Autodesk Inventor part; units mm, degrees
ref_plane "YZ Plane" through (0, 0, 0) normal (1, 0, 0) x (0, 1, 0)
ref_plane "XZ Plane" through (0, 0, 0) normal (0, 1, 0) x (-1, 0, 0)
ref_plane "XY Plane" through (0, 0, 0) normal (0, 0, 1) x (1, 0, 0)
sketch "Náčrt1" plane through (0, 0, 0) normal (0, 0, 1) x (1, 0, 0)
  line L0 (0, 0) -> (50, 0)
  line L1 (50, 0) -> (50, -50)
  line L2 (50, -50) -> (0, -50)
  line L3 (0, -50) -> (0, 0)
  dimension "d0" = 50
  dimension "d1" = 50
extrude "Vysunutí1" add sketch "Náčrt1" against normal blind 50
sketch "Náčrt2" plane through (0, 0, 0) normal (0, 1, 0) x (1, 0, 0)
  line L0 (12, 12) -> (38, 12)
  line L1 (38, 12) -> (38, 50)
  line L2 (38, 50) -> (12, 50)
  line L3 (12, 50) -> (12, 12)
  line L4 (0, 50) -> (50, 50)
  line L5 (0, 0) -> (0, 50)
  dimension "d4" = 12
  dimension "d5" = 26
  dimension "d6" = 38
extrude "Vysunutí2" cut sketch "Náčrt2" against normal blind 50
sketch "Náčrt3" plane through (50, -50, 0) normal (1, 0, 0) x (0, 0, -1)
  line L0 (12, 50) -> (37, 50)
  line L1 (37, 50) -> (37, 44)
  line L2 (37, 44) -> (12, 44)
  line L3 (12, 44) -> (12, 50)
  line L4 (0, 50) -> (50, 50)
  line L5 (0, 0) -> (0, 50)
  point P0 (37, 47)
  point P1 (12, 47)
  dimension "d9" = 12
  dimension "d10" = 25
  dimension "d11" = 6
extrude "Vysunutí3" cut sketch "Náčrt3" against normal blind 50
sketch "Náčrt4" plane through (50, -50, 0) normal (1, 0, 0) x (0, 0, -1)
  line L0 (12, 6) -> (37, 6)
  line L1 (37, 6) -> (37, 0)
  line L2 (37, 0) -> (12, 0)
  line L3 (12, 0) -> (12, 6)
  line L4 (0, 0) -> (50, 0)
  line L5 (0, 0) -> (0, 50)
  point P0 (37, 3)
  point P1 (12, 3)
  dimension "d14" = 12
  dimension "d15" = 6
  dimension "d16" = 25
extrude "Vysunutí4" cut sketch "Náčrt4" against normal blind 50
sketch "Náčrt5" plane through (50, -50, 0) normal (1, 0, 0) x (0, 0, -1)
  line L0 (50, 0) -> (50, 50)
  arc A0 (50, 0) -> (50, 50) centre (50, 25) ccw
  point P0 (0, 50)
extrude "Vysunutí5" add sketch "Náčrt5" against normal blind 50
sketch "Náčrt6" plane through (38, 0, -37) normal (0, 1, 0) x (1, 0, 0)
  line L0 (-26, 13) -> (-38, 13)
  line L1 (-26, 13) -> (0, 13)
  line L2 (0, 13) -> (0, 55.1409)
  line L3 (0, 55.1409) -> (-26, 55.1409)
  line L4 (-26, 55.1409) -> (-26, 13)
  point P0 (-38, -37)
extrude "Vysunutí6" cut sketch "Náčrt6" against normal blind 50
sketch "Náčrt7" plane through (50, -50, 0) normal (1, 0, 0) x (0, 0, -1)
  circle A0 centre (50, 25) radius 15
  point P0 (0, 50)
  dimension "d23" = 30
extrude "Vysunutí7" add sketch "Náčrt7" along normal blind 6
sketch "Náčrt8" plane through (0, -50, 0) normal (-1, 0, 0) x (0, 0, 1)
  circle A0 centre (-50, 25) radius 15
  circle A1 centre (-50, 25) radius 15
  point P0 (0, 50)
extrude "Vysunutí8" add sketch "Náčrt8" along normal blind 6
sketch "Náčrt9" plane through (-6, -25, -50) normal (-1, 0, 0) x (0, 0, 1)
  circle A0 centre (0, 0) radius 7
  point P0 (50, 25)
  dimension "d28" = 14
extrude "Vysunutí9" cut sketch "Náčrt9" against normal blind 100
sketch "Náčrt10" plane through (0, 0, 0) normal (0, 1, 0) x (1, 0, 0)
  circle A0 centre (25, -25) radius 12.5
  line L0 (0, 0) -> (13.607, -30.143)
  line L1 (50, 0) -> (50, 12)
  line L2 (50, 0) -> (36.393, -30.143)
  dimension "d31" = 25
extrude "Vysunutí10" add sketch "Náčrt10" against normal blind 50
sketch "Náčrt11" plane through (25, 0, 25) normal (0, 1, 0) x (1, 0, 0)
  point P0 (-25, 25)
sketch "Náčrt12" plane through (0, 0, 0) normal (0, 1, 0) x (1, 0, 0)
  line L0 (50, 0) -> (0, 0)
  line L1 (0, 0) -> (13.607, -30.143)
  line L2 (50, 0) -> (36.393, -30.143)
  circle A0 centre (25, -25) radius 12.5
extrude "Vysunutí11" add sketch "Náčrt12" against normal blind 12 contours L2 A0 L1 L0
sketch "Náčrt13" plane through (0, -50, 0) normal (0, -1, 0) x (1, 0, 0)
  line L0 (50, 0) -> (50, -12)
  line L1 (50, 0) -> (36.393, 30.143)
  line L2 (13.607, 30.143) -> (0, 0)
  line L3 (0, 0) -> (13.607, 30.143)
  circle A0 centre (25, 25) radius 12.5
  line L4 (50, 0) -> (50, -12)
  line L5 (0, 0) -> (0, -12)
  line L6 (50, 0) -> (0, 0)
extrude "Vysunutí12" add sketch "Náčrt13" against normal blind 12 contours L6 L2 A0 L1
sketch "Náčrt16" plane through (0, 0, 0) normal (0, 0, 1) x (1, 0, 0)
  point P0 (0, 0)
sketch "Náčrt17" plane through (0, 0, 0) normal (0, 0, 1) x (1, 0, 0)
  point P0 (0, 0)
sketch "Náčrt18" plane through (0, 0, 0) normal (0, 0, 1) x (1, 0, 0)
  line L0 (50, -10) -> (50, -40)
  line L1 (0, 0) -> (0, -50)
  line L2 (50, -19) -> (0, -19)
  line L3 (0, -19) -> (0, -31)
  line L4 (0, -31) -> (50, -31)
  line L5 (50, -31) -> (50, -19)
  dimension "d38" = 12
extrude "Vysunutí13" cut sketch "Náčrt18" along normal blind 100
sketch "Náčrt19" plane through (0, -50, -12) normal (0, -1, 0) x (1, 0, 0)
  arc A0 (13.607, 42.143) -> (36.393, 42.143) centre (25, 37) ccw
  circle A1 centre (25, 37) radius 9
  point P0 (0, 12)
  dimension "d41" = 18
extrude "Vysunutí14" cut sketch "Náčrt19" against normal blind 100
properties part number "Opakování_1" material "Stříbro"
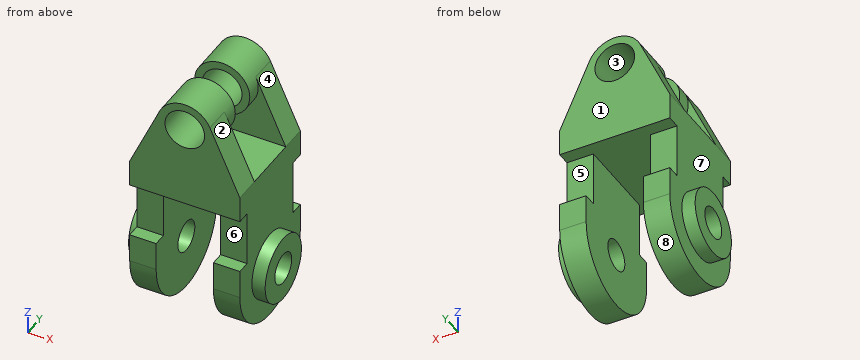
Read the model definition and answer for the solid it produces. Units are mm, in the model's axes. Face numbers are marked on the shaded views. A direction names the side the tool comes from. Round coordinates to 2 decimals unless told otherwise and drop trailing zeros. Write each loop counter-clockwise with the first axis right and the second up, starting at its lowest first coordinate (ties: lowest second). Pieces come first, ordered by that corner, then holes.
Q1. A tool of negligible diameter and unlimited length cuts with its end or side. For the marked faces 4, 5, 6, 7 and 8, from which of +Z, -Z, +X, -X, +Y, -Y can it reach the whole face along a straight path? Write none if from no direction.
Values:
face 4: +Z, +X, +Y, -Y
face 5: +X, -X, +Y
face 6: +X, -X, -Y
face 7: -X
face 8: -Z, +X, -X
Q2. Find section C-C on y = -14.5. Determine the outline of the cut face in (x, z), and give its area (3 significant figures).
Values:
outline: (-6, -60.71) - (0, -60.71) - (0, -72.69) - (12, -72.69) - (12, -12) - (38, -12) - (38, -72.69) - (50, -72.69) - (50, -60.71) - (56, -60.71) - (56, -39.29) - (50, -39.29) - (50, 0) - (0, 0) - (0, -39.29) - (-6, -39.29) - close; circle Ø25 at (25, 25); hole circle Ø18 at (25, 25)
area: 2,550 mm2
Q3. The mould has two halves that part along Z. Classify the marked faces 1, 2 and 3: released by +Z, released by -Z, zero draft, split by the parting line, or undercut.
Values:
face 1: zero draft
face 2: released by +Z
face 3: undercut
Q4. Flat-ended cylindrical pins translate along their axes: P1, Ø5, axis at x = 7.5, y = -4, coming from the +Z side; P2, Ø6, axis at x = 45.5, z = -58.5, coming from the +Y side; P3, Ø4, axis at y = -37, z = -13, coming from the -X side. Find the tip coordinate at first contact, or state that the pin passes through.
Values:
P1: stops at z = 22.15
P2: stops at y = -0.61
P3: stops at x = 0
Q5. Find section B-B on y = -25. Determine the outline of the cut face in (x, z).
Values:
outline: (-6, -65) - (0, -65) - (0, -75) - (12, -75) - (12, -57) - (-6, -57) - close; (-6, -43) - (12, -43) - (12, -12) - (38, -12) - (38, -43) - (56, -43) - (56, -35) - (50, -35) - (50, 0) - (0, 0) - (0, -35) - (-6, -35) - close; (38, -75) - (50, -75) - (50, -65) - (56, -65) - (56, -57) - (38, -57) - close
Q6. Find section D-D on z = -15. Determine the outline of the cut face in (x, y), and give its area (3 significant figures).
Values:
outline: (0, -44) - (12, -44) - (12, -6) - (0, -6) - close; (38, -44) - (50, -44) - (50, -6) - (38, -6) - close
area: 912 mm2
Q7. Find section A-A on x = 25. Determine the outline of the cut face in (y, z).
Values:
outline: (-50, -12) - (0, -12) - (0, 16) - (-19, 16) - (-19, 12.5) - (-12, 12.5) - (-12, 0) - (-38, 0) - (-38, 12.5) - (-31, 12.5) - (-31, 16) - (-50, 16) - close; (-50, 34) - (-31, 34) - (-31, 37.5) - (-50, 37.5) - close; (-19, 34) - (0, 34) - (0, 37.5) - (-19, 37.5) - close
Q8. Straight lines are drawn through the part: line 1 (Y direction, x = 5.5, z = -50); line 2 (X direction, y = -47, z = -44.5); line 3 (X direction, y = -33, z = -39). For each, find the intervals that lie inside material, in ascending order.
Values:
line 1: y = -50 to -32, -18 to 0
line 2: x = 0 to 12, 38 to 50
line 3: x = -6 to 12, 38 to 56
